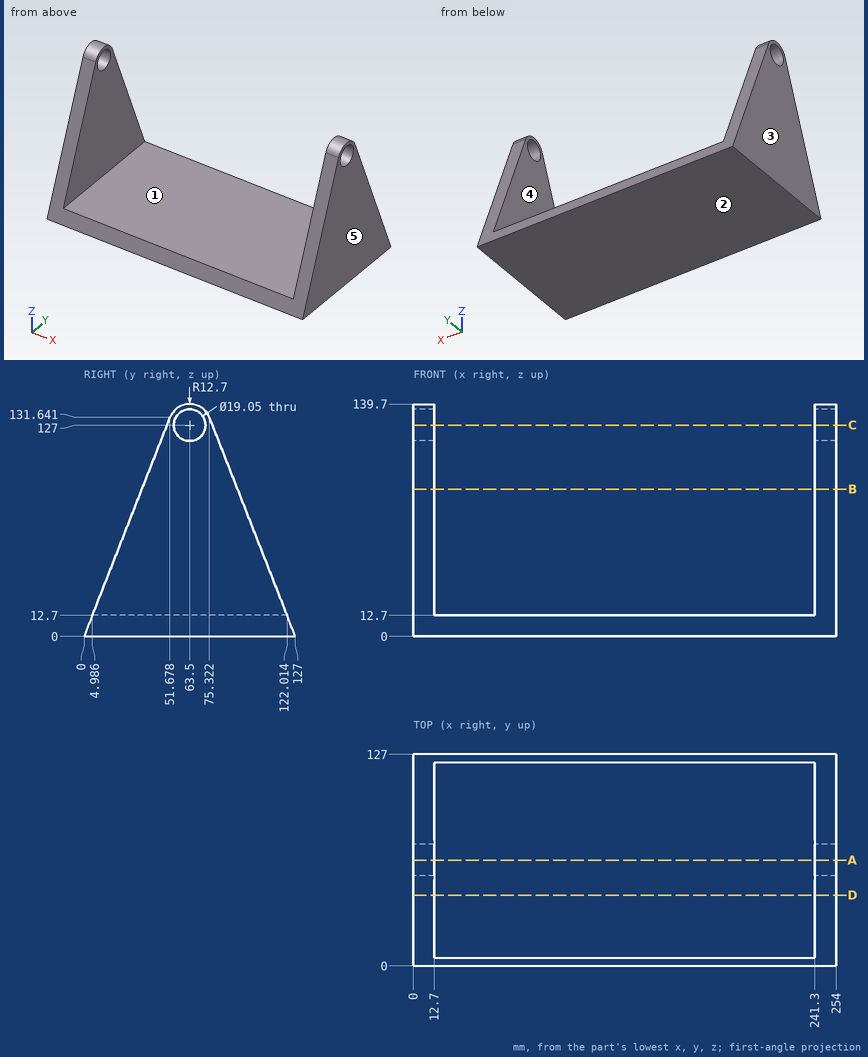
Study the drawing (mm; zero at the part's minimum x, y, z) and answer. A direction names the side the tool comes from. Round coordinates to 2 decimals unless told otherwise and drop trailing zeros. Loops run counter-clockwise (first coordinate to the right, second up) from the corner with the lowest first, then second, coordinate; pieces in that order, holes last.
Q1. Section A-A, the plane y = 63.5 is taken. Determine the outline of the cut face in (x, z) (1 decimal), then the cut area to 3 significant figures.
Q2. Section C-C, the plane z = 127 is taken. Determine the outline of the cut face in (x, y) (1 decimal).
Q3. Given pin 1 Ø3 at (x, y) = (226, 70.5) entering from +Z, flat-ended and moving along its own axis, determine where the tip first touches the part or whether it passes through.
Q4. Section B-B, the plane z = 88.5 is taken. Determine the outline of the cut face in (x, y), then the cut area to 3 significant figures.
Q5. Find the intervals of material crossed by line 1 (Z direction, x = 246, y = 63); line 2 (X direction, y = 58, z = 28); line 3 (Z direction, x = 237, y = 80.5), in increasing order.
Q6. For a pull along X with two mould halves and no side action, classify the marked faces 1, 2 and 3 as released by +X, released by -X, zero draft, split by the parting line, or undercut.
Q7. Which of the six approach directions +Z, -Z, +X, -X, +Y, -Y give full straight-line access (tool end or side, diameter ignored) to the marked faces 4 and 5?
Q8. Section D-D, the plane y = 42.5 is taken. Determine the outline of the cut face in (x, z), then the cut area to 3 significant figures.
Completed:
1. outline: (0, 0) - (254, 0) - (254, 117.5) - (241.3, 117.5) - (241.3, 12.7) - (12.7, 12.7) - (12.7, 117.5) - (0, 117.5) - close; (0, 136.5) - (12.7, 136.5) - (12.7, 139.7) - (0, 139.7) - close; (241.3, 136.5) - (254, 136.5) - (254, 139.7) - (241.3, 139.7) - close
1. area: 5,970 mm2
2. outline: (0, 49.9) - (12.7, 49.9) - (12.7, 54) - (0, 54) - close; (0, 73) - (12.7, 73) - (12.7, 77.1) - (0, 77.1) - close; (241.3, 49.9) - (254, 49.9) - (254, 54) - (241.3, 54) - close; (241.3, 73) - (254, 73) - (254, 77.1) - (241.3, 77.1) - close
3. pin 1: stops at z = 12.7
4. outline: (0, 34.74) - (12.7, 34.74) - (12.7, 92.26) - (0, 92.26) - close; (241.3, 34.74) - (254, 34.74) - (254, 92.26) - (241.3, 92.26) - close
4. area: 1,460 mm2
5. line 1: z = 0 to 117.49, 136.51 to 139.69
5. line 2: x = 0 to 12.7, 241.3 to 254
5. line 3: z = 0 to 12.7
6. face 1: undercut
6. face 2: zero draft
6. face 3: released by -X
7. face 4: +Z, +Y, -Y
7. face 5: +Z, -Z, +X, +Y, -Y
8. outline: (0, 0) - (254, 0) - (254, 108.26) - (241.3, 108.26) - (241.3, 12.7) - (12.7, 12.7) - (12.7, 108.26) - (0, 108.26) - close
8. area: 5,650 mm2
